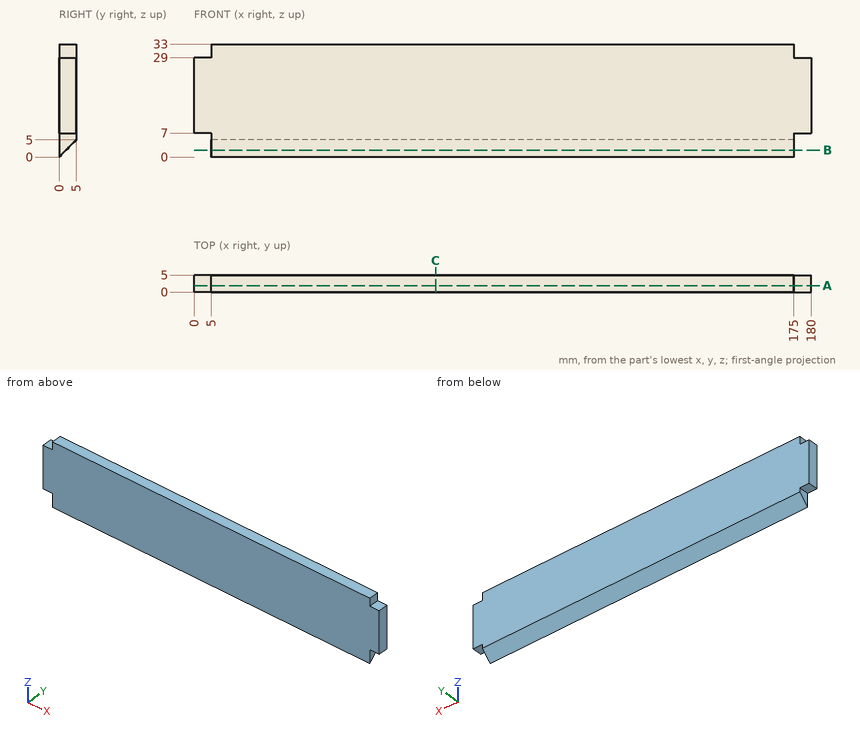
Print and shaded views of the part. All mm, measured from the part's lowest x, y and z. Give positions to 0.01 mm unless a question says otherwise; leave off trailing zeros. Write each loop counter-clockwise with the first axis right and the second up, starting at its lowest first coordinate (ties: lowest second). Pieces come first, ordered by that corner, then holes. Notation, with made-up numbers: (80.5, 86.25) - (131.5, 86.25) arc R14 ccw to (131.5, 111.25) - close; hole circle Ø6 at (33, -3.75). An arc over 180 degrees is marked (long way). Put each result on its own line as item: value.
(1) Drop flat-ended pins along their axis: pin 1 Ø1.2 at (y, z) = (3, 32) entering from +X; pin 2 Ø2.5 at (x, y) = (177.5, 3.5) entering from +Z; pin 3 Ø1.5 at (x, y) = (177.5, 2.5) entering from -Z. Give the stop position or say it passes through.
Working result:
pin 1: x = 175
pin 2: z = 29
pin 3: z = 7
(2) Wall check: L1, parallel to X at y = 2.15, z = 6; L2, parallel to Z at x = 95, y = 0.8; L3, parallel to Y at x = 37, z = 4. Give the ranges that are in metal, low to high.
Working result:
L1: 5 to 175
L2: 0.8 to 33
L3: 0 to 4
(3) Saw through at C-C (x = 70.5). List the corners of the cut face in (y, z), then the cut area to 4 significant figures.
Working result:
outline: (0, 0) - (5, 5) - (5, 33) - (0, 33) - close
area: 152.5 mm^2
(4) Saw through at A-A (y = 1.9). List the corners of the cut face in (x, z).
Working result:
outline: (0, 7) - (5, 7) - (5, 1.9) - (175, 1.9) - (175, 7) - (180, 7) - (180, 29) - (175, 29) - (175, 33) - (5, 33) - (5, 29) - (0, 29) - close
(5) Saw through at B-B (z = 2). List the corners of the cut face in (x, y), then the cut area to 3 significant figures.
Working result:
outline: (5, 0) - (175, 0) - (175, 2) - (5, 2) - close
area: 340 mm^2
